from build123d import *

# Parameters (mm, degrees)
BOSS_EXTRUDE1_DEPTH      = 1.5
BOSS_EXTRUDE1_DEPTH_BACK = 1.2
CUT_EXTRUDE1_DEPTH       = 40
SKETCH11_R               = 1
CUT_EXTRUDE2_DEPTH       = 5


with BuildPart() as part:
    # Sketch1 → Boss-Extrude1 (new body, two sides)
    with BuildSketch(Plane.XY) as boss_extrude1_sk:
        with BuildLine():
            Line((-17.999999991, 9.304537824), (-17.999999991, 10.304506021))
            Line((-17.999999991, 10.304506021), (-17.999999991, 17.303464443))
            ThreePointArc((-17.999999991, 17.303464443), (-17.707106772, 18.010571225), (-16.999999991, 18.303464443))
            Line((-16.999999991, 18.303464443), (16.999968161, 18.303464443))
            ThreePointArc((16.999968161, 18.303464443), (17.707074942, 18.010571225), (17.999968161, 17.303464443))
            Line((17.999968161, 17.303464443), (17.999968161, 9.303464443))
            Line((17.999968161, 9.303464443), (17.999968161, 6.751174458))
            ThreePointArc((17.999968161, 6.751174458), (17.707074942, 6.044067677), (16.999968161, 5.751174458))
            Line((16.999968161, 5.751174458), (16.499999991, 5.751174458))
            ThreePointArc((16.499999991, 5.751174458), (16.1464466, 5.604727849), (15.999999991, 5.251174458))
            Line((15.999999991, 5.251174458), (15.999999991, 2.751174458))
            ThreePointArc((15.999999991, 2.751174458), (15.707106772, 2.044067677), (14.999999991, 1.751174458))
            Line((14.999999991, 1.751174458), (-14.999999991, 1.751174458))
            ThreePointArc((-14.999999991, 1.751174458), (-15.707106772, 2.044067677), (-15.999999991, 2.751174458))
            Line((-15.999999991, 2.751174458), (-15.999999991, 5.251174458))
            ThreePointArc((-15.999999991, 5.251174458), (-16.1464466, 5.604727849), (-16.499999991, 5.751174458))
            Line((-16.499999991, 5.751174458), (-16.999999991, 5.751174458))
            ThreePointArc((-16.999999991, 5.751174458), (-17.707106772, 6.044067677), (-17.999999991, 6.751174458))
            Line((-17.999999991, 6.751174458), (-17.999999991, 9.304537824))
        make_face()
    extrude(amount=BOSS_EXTRUDE1_DEPTH)
    extrude(boss_extrude1_sk.sketch, amount=-BOSS_EXTRUDE1_DEPTH_BACK)

    # Sketch3 → Cut-Extrude1 (cut)
    with BuildSketch(Plane(origin=(17.999968161, 0, 0), x_dir=(0, 0, -1), z_dir=(1, 0, 0))):
        with BuildLine():
            Line((0.023796664, 6.751174458), (0.023796664, 5.754537824))
            ThreePointArc((0.023796664, 5.754537824), (0.053060483, 3.748723952), (0.23729316, 1.751174458))
            Line((0.23729316, 1.751174458), (1.2708887, 1.751174458))
            Line((1.2708887, 1.751174458), (1.2708887, 10.304537824))
            Line((1.2708887, 10.304537824), (1.2708887, 10.30507849))
            ThreePointArc((1.2708887, 10.30507849), (7.212872074, 16.614024598), (1.023796664, 22.680762846))
            Line((1.023796664, 22.680762846), (1.023796664, 17.303464443))
            Line((1.023796664, 17.303464443), (1.2, 17.303464443))
            Line((1.2, 17.303464443), (1.2, 6.751174458))
            Line((1.2, 6.751174458), (0.023796664, 6.751174458))
        make_face()
        Polygon((0.023796664, 10.304537824), (0.023796664, 6.751174458), (1.2, 6.751174458), (1.2, 17.303464443), (1.023796664, 17.303464443), (1.023796664, 10.304537824), align=None)
        with BuildLine():
            ThreePointArc((-1.485404738, 6.692099607), (-1.491731963, 6.721473521), (-1.496283327, 6.751174458))
            Line((-1.496283327, 6.751174458), (-1.5, 6.751174458))
            Line((-1.5, 6.751174458), (-1.5, 1.751174458))
            Line((-1.5, 1.751174458), (0.126821568, 1.751174458))
            ThreePointArc((0.126821568, 1.751174458), (-0.181429151, 1.857497567), (-0.358583171, 2.131248481))
            Line((-0.358583171, 2.131248481), (-1.485404738, 6.692099607))
        make_face()
        with BuildLine():
            Line((-1.5, 6.751174458), (-1.496283327, 6.751174458))
            ThreePointArc((-1.496283327, 6.751174458), (-1.499069967, 6.781543322), (-1.5, 6.812025585))
            Line((-1.5, 6.812025585), (-1.5, 6.751174458))
        make_face()
    extrude(amount=-CUT_EXTRUDE1_DEPTH, mode=Mode.SUBTRACT)

    # Sketch11 → Cut-Extrude2 (cut)
    with BuildSketch(Plane(origin=(0, 0, -1.023796664), x_dir=(-1, 0, 0), z_dir=(0, 0, -1))):
        with Locations((11.000015915, 15.294537824)):
            Circle(SKETCH11_R)
        with Locations((-10.999984085, 15.294537824)):
            Circle(SKETCH11_R)
    extrude(amount=-CUT_EXTRUDE2_DEPTH, mode=Mode.SUBTRACT)


solid = part.part
Could you check a few things on this model? Use its own coordinates, in mm. A direction names the side the tool comes from. Give positions to 0.01 mm unless a question says otherwise; leave off trailing zeros. Write each loop counter-clockwise with the first axis right and the second up, starting at its lowest first coordinate (ties: lowest second). Pieces come first, ordered by that corner, then holes. Notation, with made-up numbers: (-0.5, 65.5) -> (10.5, 65.5) arc R17 ccw to (10.5, 70.5) -> close; hole circle Ø11 at (12, -17.5). An arc over 180 degrees is marked (long way). Write each question's results on one line, items separated by ' | '. Start each with the question number.
Q1. Suppose I cut it at A-A, the plane x = 11. List the corners of the cut face in (y, z) for me, and give its area (3 significant figures).
Q2. We'd pull the mould along Y, two halves only. Please class faces 4 (the face through (-17.715, 18.003, 0.256)), 5 (the face through (-16, 4, 0.4)), 6 (the face through (17.715, 6.052, 0.747)), 7 (the face through (0.24, 3.78, -0.05)): +Y half, -Y half, draft (parallel to the pull), parting line (faces both ways), or undercut.
Q3. I need wall thicknesses on probe 1 along Y at (x, z) = (-3, -0.4); probe 2 along X at (y, z) = (16, -0.65); probe 3 along Y at (x, z) = (10.5, -0.8). Which ranges of each line are inside material? Lowest first, please.
Q4. Suppose I cut it at B-B, the plane x = 4. List the corners of the cut face in (y, z) for me.
Q5. I'm going to push flat-ended pins straight in: pin 1 Ø1.4 at (x, y) = (9, 9) entering from -Z; pin 2 Ø0.6 at (x, z) = (-17, 0.5) entering from -Y; pin 3 Ø1.2 at (x, y) = (-11, 15.29) entering from +Z. Where does each tip first touch, or does it pass through?
Q6. Suppose I cut it at D-D, the plane y = 7.75. List the corners of the cut face in (x, z) for me, and give its area (3 significant figures).
Q7. Which directions (+Z, -Z, +X, -X, +Y, -Y) give clear straight access to the entire face, cutting with the end or side of a thin tool? Please do faces 1 (the face through (18, 13, 0)), 2 (the face through (16, 4, 0.4)), 3 (the face through (0, 8, -0.024)).
Q8. Suppose I cut it at C-C, the plane y = 14.75. List the corners of the cut face in (x, z) for me, and give its area (3 significant figures).
Outcome:
1) outline: (1.75, -0.24) arc R25.93 cw to (5.75, -0.02) -> (10.3, -0.02) -> (10.3, -1.02) -> (14.29, -1.02) -> (14.29, 1.5) -> (6.81, 1.5) arc R0.5 ccw to (6.69, 1.49) -> (2.13, 0.36) arc R0.5 ccw to (1.75, -0.13) -> close; (16.29, -1.02) -> (18.3, -1.02) -> (18.3, 1.5) -> (16.29, 1.5) -> close | area: 25.3 mm2
2) face 4: +Y half | face 5: draft | face 6: -Y half | face 7: undercut
3) probe 1: 10.3 to 18.3 | probe 2: -18 to -11.71, -10.29 to 10.29, 11.71 to 18 | probe 3: 10.3 to 14.43, 16.16 to 18.3
4) outline: (1.75, -0.24) arc R25.93 cw to (5.75, -0.02) -> (10.3, -0.02) -> (10.3, -1.02) -> (18.3, -1.02) -> (18.3, 1.5) -> (6.81, 1.5) arc R0.5 ccw to (6.69, 1.49) -> (2.13, 0.36) arc R0.5 ccw to (1.75, -0.13) -> close
5) pin 1: z = -0.02 | pin 2: y = 5.75 | pin 3: through
6) outline: (-18, -0.02) -> (18, -0.02) -> (18, 1.5) -> (-18, 1.5) -> close | area: 54.9 mm2
7) face 1: +Z, -Z, +X, +Y, -Y | face 2: +Z, -Z, +X, -Y | face 3: -Z, +X, -X
8) outline: (-18, -1.02) -> (-11.84, -1.02) -> (-11.84, 1.5) -> (-18, 1.5) -> close; (-10.16, -1.02) -> (10.16, -1.02) -> (10.16, 1.5) -> (-10.16, 1.5) -> close; (11.84, -1.02) -> (18, -1.02) -> (18, 1.5) -> (11.84, 1.5) -> close | area: 82.4 mm2
